Can you work these out from the drawing? Everything is in mm from the part's minimum corner. A direction names the side the tool comes from. Round coordinates to 2 decimals unless told otherwise and drop trailing zeros. Write each loop counter-clockwise with the first axis right and the second up, starting at its lowest first coordinate (ties: lowest second). Pieces come first, ordered by that corner, then holes. Notation, with made-up numbers: (70, 36) - (129, 36) arc R21 ccw to (129, 72) - close; hole circle Ø10 at (-6.5, 6.5). An arc over 180 degrees is marked (long way). Write each question's results on one line, items separated by ' | '. Start each with the question number.
(1) Imagine slicing it at C-C on x = 8.25. Write out the boundary of the cut face in (y, z) (1 decimal), then the cut area to 3 significant figures.
(2) Imagine slicing it at A-A on z = 8. Write out the boundary of the cut face in (x, y) (1 decimal).
(3) On a 3-axis mill with a long thin cutter (end or side, diameter ignored), from which of +Z, -Z, +X, -X, +Y, -Y can I reach the whole of each face in a straight line? I mean the marked faces 1, 2, 3 and 4. Say none if no direction works.
(4) Please list where these lines run through material, in increasing order: line 1 (Y direction, x = 15, z = 2.5) (1 decimal); line 2 (X direction, y = 21, z = 2.25) (1 decimal); line 3 (X direction, y = 6, z = 4). Write a range as [from, to].
(5) Imagine slicing it at B-B on y = 9.25. Write out the boundary of the cut face in (x, z).
(6) For P1, Ø1.3, axis at y = 9, z = 6.5, coming from the -X side; P2, Ø1.6, axis at y = 1, z = 5.5, coming from the +X side; P3, Ø0.5, axis at x = 6, z = 9, coming from the +Y side, each with a flat end and sliding along its axis, tell me the tip position at first contact or that it passes through.
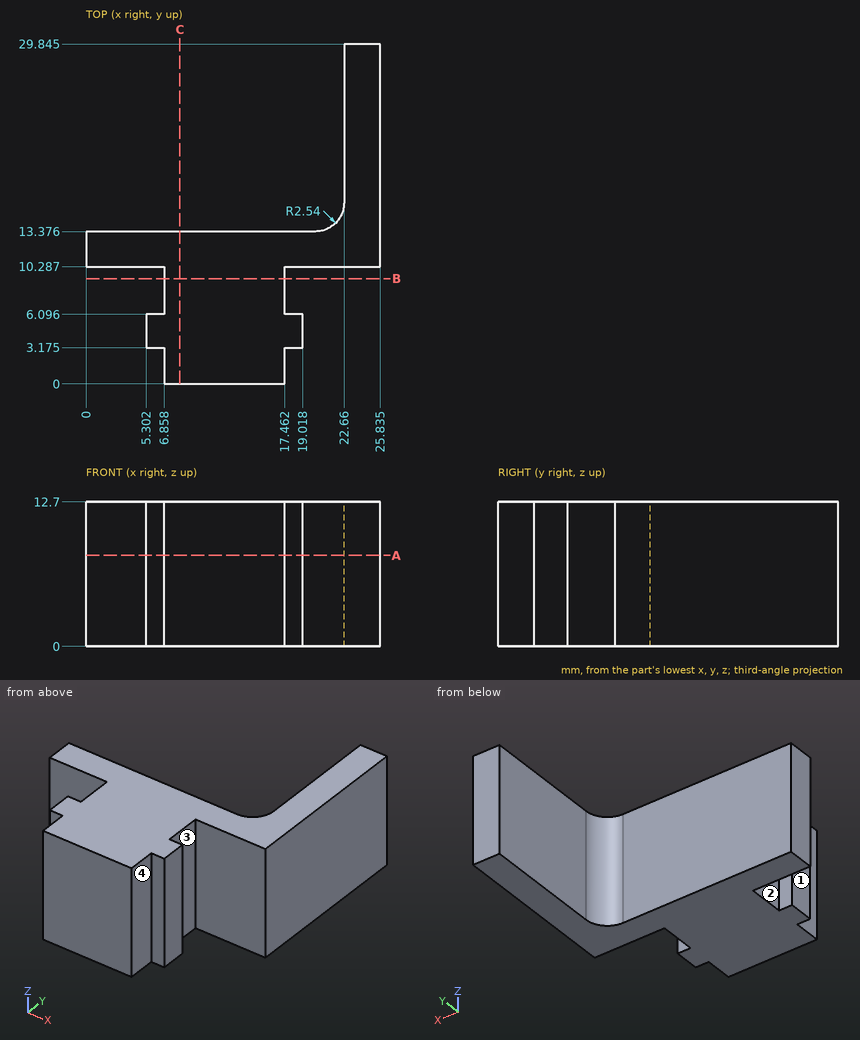
Response:
1) outline: (0, 0) - (13.4, 0) - (13.4, 12.7) - (0, 12.7) - close | area: 170 mm²
2) outline: (0, 10.3) - (6.9, 10.3) - (6.9, 6.1) - (5.3, 6.1) - (5.3, 3.2) - (6.9, 3.2) - (6.9, 0) - (17.5, 0) - (17.5, 3.2) - (19, 3.2) - (19, 6.1) - (17.5, 6.1) - (17.5, 10.3) - (25.8, 10.3) - (25.8, 29.8) - (22.7, 29.8) - (22.7, 15.9) arc R2.5 cw to (20.1, 13.4) - (0, 13.4) - close
3) face 1: +Z, -Z, -X, -Y | face 2: +Z, -Z, -X | face 3: +Z, -Z, +X | face 4: +Z, -Z, +X, -Y
4) line 1: [0, 13.4] | line 2: [22.7, 25.8] | line 3: [5.3, 19.02]
5) outline: (6.86, 0) - (17.46, 0) - (17.46, 12.7) - (6.86, 12.7) - close
6) P1: x = 6.86 | P2: x = 17.46 | P3: y = 13.38
